For this review, take the finished solid that the model builds, in its own axes (mm). Face numbers are marked on the shaded views. Give positions to 0.01 mm unless a question says otherwise; leave off trailing zeros. Write each loop counter-clockwise with the first axis right and the second up, starting at its lowest first coordinate (ties: lowest second). Pieces come first, ordered by that corner, then holes.
Q1. Mouldability with a two-part tool opening along X and no side actions: class the marked faces 1 and 2 as released by +X, released by -X, zero draft, split by the parting line, or undercut.
Q2. We need section D-D (x = -16). Write out the cut boundary in (y, z).
Q3. Insertion check: P1, Ø1, axis at y = 4, z = -43.5, coming from the +X side; P2, Ø2.5, axis at x = -41, y = 2, coming from the -Z side; P3, Ø0.9, axis at x = 5.5, y = 3.5, coming from the -Z side. Each pin has a flat end and moves straight along its axis. Give the tip position at first contact, or say it passes through.
Q4. We need section B-B (x = -48). Write out the cut boundary in (y, z), then the cut area to 3 significant figures.
Q5. We need section A-A (z = -11). Write out the cut boundary in (x, y).
Q6. We need section C-C (y = 3.15). Give the number of separate pieces and of enclosed holes in the cut face, then the cut area to 3 significant figures.
Q7. For line 1 (X direction, y = 1.9, z = 0.5); line 2 (X direction, y = 2.8, z = 10); line 3 (X direction, y = 0.75, z = -27), list the stretches that pass through material, from the lowest coordinate up.
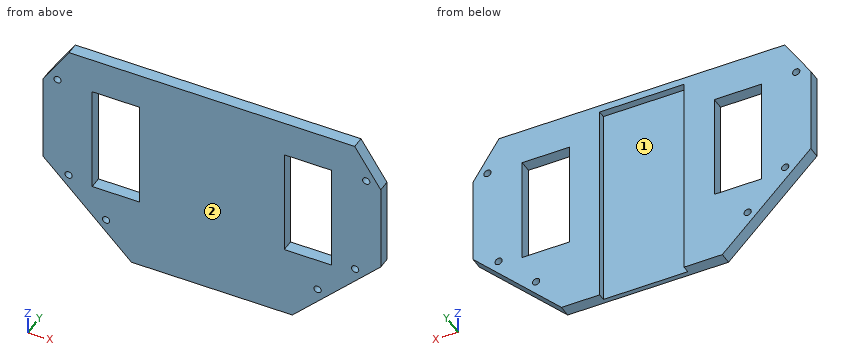
```python
from build123d import *

# Parameters (mm, degrees)
SKETCH1_R           = 1.5
SKETCH1_W           = 19.6
SKETCH1_H           = 45.1
BOSS_EXTRUDE1_DEPTH = 5
SKETCH2_W           = 35
SKETCH2_H           = 87
CUT_EXTRUDE1_DEPTH  = 3


with BuildPart() as part:
    # Sketch1 → Boss-Extrude1 (new body)
    with BuildSketch(Plane(origin=(0, 0, 0), x_dir=(1, 0, 0), z_dir=(0, 1, 0))):
        Polygon((-59.213749531, -30), (-70, -13.390630812), (-70, 23.338095117), (-33.338095117, 60), (0, 60), (0, -30), align=None)
        with Locations((-43.840620434, 43.840620434)):
            Circle(SKETCH1_R, mode=Mode.SUBTRACT)
        with Locations((-59.39696962, 28.284271247)):
            Circle(SKETCH1_R, mode=Mode.SUBTRACT)
        with Locations((-63.979633983, -15.316867676)):
            Circle(SKETCH1_R, mode=Mode.SUBTRACT)
        with Locations((-39.8, 7.55)):
            Rectangle(SKETCH1_W, SKETCH1_H, mode=Mode.SUBTRACT)
    boss_extrude1 = extrude(amount=BOSS_EXTRUDE1_DEPTH)

    # Mirror1: Boss-Extrude1 across plane
    add(boss_extrude1.mirror(Plane(origin=(0, 5, 30), x_dir=(0, 0, 1), z_dir=(-1, 0, 0))))

    # Sketch2 → Cut-Extrude1 (cut)
    with BuildSketch(Plane(origin=(0, 5, 0), x_dir=(1, 0, 0), z_dir=(0, 1, 0))):
        with Locations((0, 16.5)):
            Rectangle(SKETCH2_W, SKETCH2_H)
    extrude(amount=-CUT_EXTRUDE1_DEPTH, mode=Mode.SUBTRACT)


solid = part.part
```
Computed:
1. face 1: undercut
1. face 2: zero draft
2. outline: (0, -60) - (2, -60) - (2, 27) - (5, 27) - (5, 30) - (0, 30) - close
3. P1: stops at x = 50.34
3. P2: stops at z = -53.59
3. P3: stops at z = 27
4. outline: (0, -45.34) - (5, -45.34) - (5, -30.1) - (0, -30.1) - close; (0, 15) - (5, 15) - (5, 30) - (0, 30) - close
4. area: 151 mm2
5. outline: (-70, 0) - (-49.6, 0) - (-49.6, 5) - (-70, 5) - close; (-30, 0) - (30, 0) - (30, 5) - (17.5, 5) - (17.5, 2) - (-17.5, 2) - (-17.5, 5) - (-30, 5) - close; (49.6, 0) - (70, 0) - (70, 5) - (49.6, 5) - close
6. separate pieces: 1
6. enclosed holes: 8
6. area: 6,220 mm2
7. line 1: x = -70 to -49.6, -30 to 30, 49.6 to 70
7. line 2: x = -70 to -49.6, -30 to -17.5, 17.5 to 30, 49.6 to 70
7. line 3: x = -66.34 to -60.17, -58.62 to -49.6, -30 to 30, 49.6 to 58.62, 60.17 to 66.34
